Part model, mm, in its own coordinate system. A direction names the side the tool comes from. Give positions to 0.01 mm unless a question says otherwise; leave off trailing zeros. Order: outer loops, then holes, each group sorted by start corner. A loop starts at its lowest first (then second) coordinate and runs counter-clockwise, first axis right, second up. Notation, with made-up numbers: M -19.5,29.25 L 16.5,29.25 A25 cw 16.5,44.25 Z; hole C 66.25,72 d2. An arc over 180 degrees is marked long. One line per question, with ' | ' between items.
Autodesk Inventor part; units mm, degrees
ref_plane "YZ Plane" through (0, 0, 0) normal (1, 0, 0) x (0, 1, 0)
ref_plane "XZ Plane" through (0, 0, 0) normal (0, 1, 0) x (-1, 0, 0)
ref_plane "XY Plane" through (0, 0, 0) normal (0, 0, 1) x (1, 0, 0)
sketch "スケッチ1" plane through (0, 0, 0) normal (1, 0, 0) x (0, 1, 0)
  line L0 (0, 0) -> (15.2, 0)
  line L1 (15.2, 0) -> (15.2, -62.0281)
  line L2 (15.2, -62.0281) -> (0, -62.0281)
  line L3 (0, -62.0281) -> (0, 0)
  circle A0 centre (-15, -24.3937) radius 1.6
  circle A1 centre (-25, -24.3937) radius 1.6
  circle A2 centre (-15, -37.3937) radius 1.6
  circle A3 centre (-25, -37.3937) radius 1.6
  line L4 (25.2, -19.3937) -> (-10, -19.3937)
  line L5 (-10, -19.3937) -> (-10, -42.3937)
  line L6 (-10, -42.3937) -> (25.2, -42.3937)
  line L7 (25.2, -42.3937) -> (25.2, -19.3937)
  line L8 (-10, -19.3937) -> (-30, -19.3937)
  line L9 (-30, -19.3937) -> (-30, -42.3937)
  line L10 (-30, -42.3937) -> (-10, -42.3937)
  line L11 (-10, -42.3937) -> (-10, -19.3937)
  point P0 (0, -42.3937)
  point P1 (0, -19.3937)
  point P2 (15.2, -19.3937)
  point P3 (15.2, -42.3937)
  point P4 (-10, -42.3937)
  dimension "d0" = 15.2
  dimension "d1" = 3.2
  dimension "d2" = 3.2
  dimension "d3" = 3.2
  dimension "d4" = 3.2
  dimension "d5" = 10
  dimension "d6" = 10
  dimension "d7" = 13
  dimension "d8" = 13
  dimension "d9" = 0
  dimension "d10" = 0
  dimension "d12" = 10
  dimension "d13" = 10
  dimension "d14" = 5
  dimension "d15" = 5
  dimension "d16" = 5
  dimension "d17" = 0
  dimension "d18" = 5
extrude "押し出し1" add sketch "スケッチ1" against normal blind 25 contours L3 L6 L5 L4 | L4 L7 L6 L1
extrude "押し出し2" add sketch "スケッチ1" along normal blind 10 contours L4 L1 L6 L3 | L3 L6 L5 L4 | L4 L7 L6 L1 | L5 L10 L9 L8
sketch "スケッチ2" plane through (-25, 25.2, -19.3937) normal (0, 1, 0) x (1, 0, 0)
  line L0 (25, 23) -> (0, 23)
  line L1 (5, 23) -> (5, 0)
  line L2 (25, 0) -> (0, 0)
  line L3 (0, 0) -> (0, 23)
  point P0 (25, -19.3937)
  point P1 (5, 11.5)
  dimension "d23" = 5
hole "穴1" at (-20, 25.2, -30.8937) direction (0, -1, 0) diameter 3.2 end through all
fillet "フィレット1" radius 2 6 edges at (-25, 20.2, -19.3937) (-25, -5, -19.3937) (-25, -5, -42.3937) (-25, 20.2, -42.3937) (5, -30, -19.3937) (5, -30, -42.3937)
equation "\"d6\" = d5"
equation "\"d8\" = d7"
properties part number "dribl-v1-3DP-cc-f-1" material "ABS プラスチック"
1. Mould opens along X. For faces 4 (the cylindrical face through (-20.07, -5.07, -32.492)), 5 (the flat face through (-25, -5, -31)), 6 (the flat face through (10, -3, -31)), 7 (the cylindrical face through (-20.07, 20.13, -32.492)) say: released by +X, released by -X, zero draft, split by the parting line, or undercut.
Worked out:
face 4: undercut | face 5: released by -X | face 6: released by +X | face 7: undercut
2. Tool access for faces 1 (the flat face through (-25, 20, -31)), 2 (the flat face through (0, 7, -31)), 3 (the flat face through (-12, -10, -31)): list every direction of +Z, -Z, +X, -X, +Y, -Y with a clear straight run to the whole face (end or side of a thin tool).
Worked out:
face 1: +Z, -Z, -X, +Y, -Y | face 2: +Z, -Z, -X | face 3: +Z, -Z, -X, -Y
3. Probe L1, parallel to Y at x = -15, z = -22.75; L2, parallel to Y at x = 4, z = -36.25; L3, parallel to Z at x = -20, y = 22.5. List the from-to ranges inside material, lowest first. Write a range as from..to.
Worked out:
L1: y = -10..0, 15.2..25.2 | L2: y = -30..-26.12, -23.88..-16.12, -13.88..25.2 | L3: z = -42.39..-32.49, -29.29..-19.39
4. Slice it at C-C on y = -25. Give the cut face in (x, z).
Worked out:
outline: M 0,-42.39 L 10,-42.39 L 10,-38.99 L 0,-38.99 Z; M 0,-35.79 L 10,-35.79 L 10,-25.99 L 0,-25.99 Z; M 0,-22.79 L 10,-22.79 L 10,-19.39 L 0,-19.39 Z
5. Slice it at B-B on x = -20. Give the cut face in (y, z), then the cut area to 3 significant figures.
Worked out:
outline: M -10,-42.39 L 0,-42.39 L 0,-32.49 L -10,-32.49 Z; M -10,-29.29 L 0,-29.29 L 0,-19.39 L -10,-19.39 Z; M 15.2,-42.39 L 25.2,-42.39 L 25.2,-32.49 L 15.2,-32.49 Z; M 15.2,-29.29 L 25.2,-29.29 L 25.2,-19.39 L 15.2,-19.39 Z | area: 396 mm2
6. Slice it at A-A on x = -7. Give the cut face in (y, z), then the cut area to 3 significant figures.
Worked out:
outline: M -10,-42.39 L 0,-42.39 L 0,-19.39 L -10,-19.39 Z; M 15.2,-42.39 L 25.2,-42.39 L 25.2,-19.39 L 15.2,-19.39 Z | area: 460 mm2
7. Slice it at D-D on z = -38.25. Give the cut face in (x, y), then the cut area to 3 significant figures.
Worked out:
outline: M -25,-10 L 0,-10 L 0,-13.65 L 10,-13.65 L 10,25.2 L -25,25.2 L -25,15.2 L 0,15.2 L 0,0 L -25,0 Z; M 0,-30 L 10,-30 L 10,-26.35 L 0,-26.35 Z; M 0,-23.65 L 10,-23.65 L 10,-16.35 L 0,-16.35 Z | area: 998 mm2
8. Drop flat-ended pins along their axis: pin 1 (3 mm diameter, centred on x = -6, z = -33.5, fed in from -Y); pin 2 (7.5 mm diameter, centred on y = 8, z = -33.5, fed in from -X). Give the stop position or say it passes through.
Worked out:
pin 1: stops at y = -10 | pin 2: stops at x = 0
